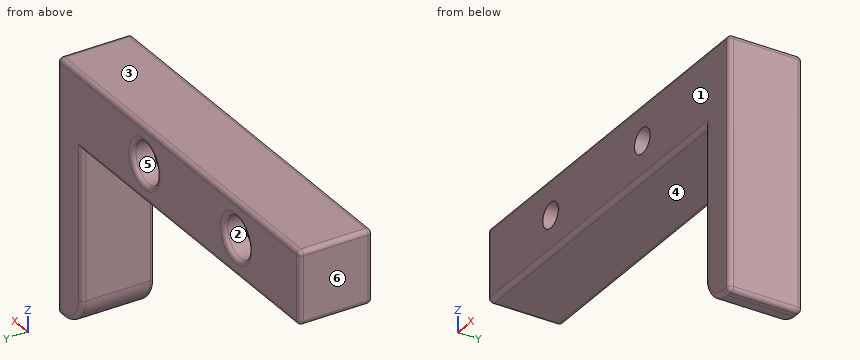
```python
from build123d import *

# Parameters (mm, degrees)
SKETCH1_W           = 60.325
SKETCH1_H           = 12.7
SKETCH1_R           = 2.159
BOSS_EXTRUDE1_DEPTH = 12.7
SKETCH5_W           = 43.775259309
SKETCH5_H           = 12.7
BOSS_EXTRUDE3_DEPTH = 6.604
SKETCH6_R           = 3.556
CUT_EXTRUDE1_DEPTH  = 3.81
FILLET2_R           = 5.08
FILLET3_R           = 0.762


with BuildPart() as part:
    # Sketch1 → Boss-Extrude1 (new body)
    with BuildSketch(Plane(origin=(0, 0, 0), x_dir=(1, 0, 0), z_dir=(0, 1, 0))):
        with Locations((30.1625, 6.35)):
            Rectangle(SKETCH1_W, SKETCH1_H)
        with Locations((17.4625, 6.35)):
            Circle(SKETCH1_R, mode=Mode.SUBTRACT)
        with Locations((42.8625, 6.35)):
            Circle(SKETCH1_R, mode=Mode.SUBTRACT)
    extrude(amount=BOSS_EXTRUDE1_DEPTH)

    # Sketch5 → Boss-Extrude3 (add)
    with BuildSketch(Plane(origin=(60.325, 0, 0), x_dir=(0, 0, -1), z_dir=(1, 0, 0))):
        with Locations((21.887629655, 6.35)):
            Rectangle(SKETCH5_W, SKETCH5_H)
    extrude(amount=BOSS_EXTRUDE3_DEPTH)

    # Sketch6 → Cut-Extrude1 (cut)
    with BuildSketch(Plane(origin=(0, 12.7, 0), x_dir=(1, 0, 0), z_dir=(0, 1, 0))):
        with Locations((42.8625, 6.35)):
            Circle(SKETCH6_R)
        with Locations((17.4625, 6.35)):
            Circle(SKETCH6_R)
    extrude(amount=-CUT_EXTRUDE1_DEPTH, mode=Mode.SUBTRACT)

    # Fillet2
    fillet2_edges = [part.edges().sort_by_distance(p)[0] for p in [
        (60.325, 6.35, -43.775259309),
    ]]
    fillet(fillet2_edges, radius=FILLET2_R)

    # Fillet3
    fillet3_edges = [part.edges().sort_by_distance(p)[0] for p in [
        (30.1625, 12.7, -12.7),
        (60.325, 0, -25.697629654),
        (66.167, 0, -43.775259309),
        (66.167, 12.7, -43.775259309),
        (66.929, 6.35, 0),
        (66.929, 0, -21.887629654),
        (66.929, 6.35, -43.775259309),
        (66.929, 12.7, -21.887629654),
        (39.3065, 12.7, -6.35),
        (0, 12.7, -6.35),
        (13.9065, 12.7, -6.35),
        (30.1625, 0, -12.7),
        (60.325, 12.7, -25.697629654),
        (61.812897552, 12.7, -42.287361757),
        (61.812897552, 0, -42.287361757),
        (33.4645, 0, 0),
        (0, 0, -6.35),
        (33.4645, 12.7, 0),
        (0, 6.35, -12.7),
        (0, 6.35, 0),
    ]]
    fillet(fillet3_edges, radius=FILLET3_R)


solid = part.part
```
The listing builds one solid part. Answer for the finished solid, in the listing's coordinates (mm). Face numbers are marked on the shaded views. A direction names the side the tool comes from. Coordinates: 2 decimals unless noted, no trailing zeros. Order: outer loops, then holes, each group sorted by start corner. A loop starts at its lowest first (then second) coordinate and runs counter-clockwise, first axis right, second up. Notation, with made-up numbers: M -10,27.25 L 32,27.25 A10 cw 32,40.25 Z; hole C -20,55.25 d7. An arc over 180 degrees is marked long. Answer as a JSON object with one key per item and string values. Group by question number.
1. Flat-ended cylindrical pins translate along their axes: P1, Ø1, axis at x = 13.5, y = 5, coming from the -Z side; P2, Ø2, axis at y = 2.5, z = -30.5, coming from the -X side (3 decimals); P3, Ø4, axis at x = 42.86, z = -6.35, coming from the +Y side; P4, Ø3.5, axis at x = 18.5, z = -5.5, coming from the +Y side. Find the tip coordinate at first contact, or state that the pin passes through.
2. Section D-D on z = -30 is taken. Write down the section's boundary in (x, y) (3 decimals).
3. Section C-C on x = 12 is taken. Write down the section's boundary in (y, z).
4. Determine the mould class of the marked faces 1, 2 and 3 for opening direction Z: released by +Z, released by -Z, zero draft, split by the parting line, or undercut.
5. Straight lines are drawn through the part: line 1 (X direction, y = 10.45, z = -6.35); line 2 (X direction, y = 2, z = -6.35); line 3 (Y direction, x = 61, z = -29). For each, find the intervals that lie inside material, in ascending order.
6. Section B-B on y = 1.5 is taken. State how many separate pieces and enclosed holes the cut face has, then the cut area to 3 significant figures.
7. Section A-A on z = -6.35 is taken. Write down the section's boundary in (x, y), then the cut area to 3 significant figures.
8. A tool of negligible diameter and unlimited length cuts with its end or side. For the marked faces 4, 5 and 6, from which of +Z, -Z, +X, -X, +Y, -Y can it reach the whole face along a straight path? Write none if from no direction.
Values follow:
{
 "1": {"P1": "z = -12.7", "P2": "x = 60.325", "P3": "through", "P4": "y = 8.89"},
 "2": {"outline": "M 60.325,0.762 A0.762 ccw 61.087,0 L 66.167,0 A0.762 ccw 66.929,0.762 L 66.929,11.938 A0.762 ccw 66.167,12.7 L 61.087,12.7 A0.762 ccw 60.325,11.938 Z"},
 "3": {"outline": "M 0,-11.94 A0.76 ccw 0.76,-12.7 L 11.94,-12.7 A0.76 ccw 12.7,-11.94 L 12.7,-0.76 A0.76 ccw 11.94,0 L 0.76,0 A0.76 ccw 0,-0.76 Z"},
 "4": {"face 1": "zero draft", "face 2": "undercut", "face 3": "released by +Z"},
 "5": {"line 1": "0 to 13.91, 21.02 to 39.31, 46.42 to 66.93", "line 2": "0 to 15.3, 19.62 to 40.7, 45.02 to 66.93", "line 3": "0 to 12.7"},
 "6": {"separate pieces": "1", "enclosed holes": "2", "area": "1,020 mm2"},
 "7": {"outline": "M 0,0.76 A0.76 ccw 0.76,0 L 15.3,0 L 15.3,8.89 L 13.91,8.89 L 13.91,11.94 A0.76 ccw 13.14,12.7 L 0.76,12.7 A0.76 ccw 0,11.94 Z; M 19.62,0 L 40.7,0 L 40.7,8.89 L 39.31,8.89 L 39.31,11.94 A0.76 ccw 38.54,12.7 L 21.78,12.7 A0.76 ccw 21.02,11.94 L 21.02,8.89 L 19.62,8.89 Z; M 45.02,0 L 66.17,0 A0.76 ccw 66.93,0.76 L 66.93,11.94 A0.76 ccw 66.17,12.7 L 47.18,12.7 A0.76 ccw 46.42,11.94 L 46.42,8.89 L 45.02,8.89 Z", "area": "718 mm2"},
 "8": {"face 4": "-Z, -X, +Y, -Y", "face 5": "+Y", "face 6": "+Z, -Z, -X, +Y, -Y"}
}
